Check sheet for the drawn part. Datum: minimum x, y, z corner. Units: mm. A direction names the side the tool comes from. Coordinates: 2 decimals unless noted, no trailing zeros. Write each loop counter-clockwise with the first axis right and the second up, starting at its lowest first coordinate (ties: lowest second). Pieces come first, ordered by that corner, then holes. Notation, with made-up numbers: (89.5, 6) -> (129.5, 6) arc R29 cw to (129.5, 37) -> close; hole circle Ø6 at (40, 83.5). An arc over 180 degrees is marked (long way). Answer in a Markdown table with one row per item. Add a question column.
Q1. Section check B-B, the plane y = 7. Record the boundary of the cut face in (x, z), and give its area (3 significant figures).
Q2. Gauge pin test, flat ends, axial feed: P1, Ø1, axis at y = 3, z = 22, coming from the +X side; P2, Ø3, axis at x = 6, z = 21.5, coming from the +Y side; P3, Ø0.8, axis at y = 7, z = 25.5, coming from the +X side; P4, Ø6, axis at x = 13.5, y = 10.5, coming from the +Z side. Record the tip position at first contact, or that the pin passes through.
Q3. Section check C-C, the plane x = 13. Record the boundary of the cut face in (y, z).
Q4. Section check D-D, the plane y = 9. Record the boundary of the cut face in (x, z), and give its area (3 significant figures).
Q5. Tool access check on the marked faces 1, 2 and 3. Record the directions out of +Z, -Z, +X, -X, +Y, -Y that give a thin tool (end or side, any length) a straight path to the whole face; none if there is none.
Q6. Thickness scan on line 1 (Y direction, x = 22.5, z = 14.25); line 2 (X direction, y = 5.75, z = 16.5); line 3 (Z direction, x = 16.25, y = 5). Record the ranges inside material, lowest first.
Q7. Section check A-A, the plane z = 25.75. Record the boundary of the cut face in (x, y), and give its area (3 significant figures).
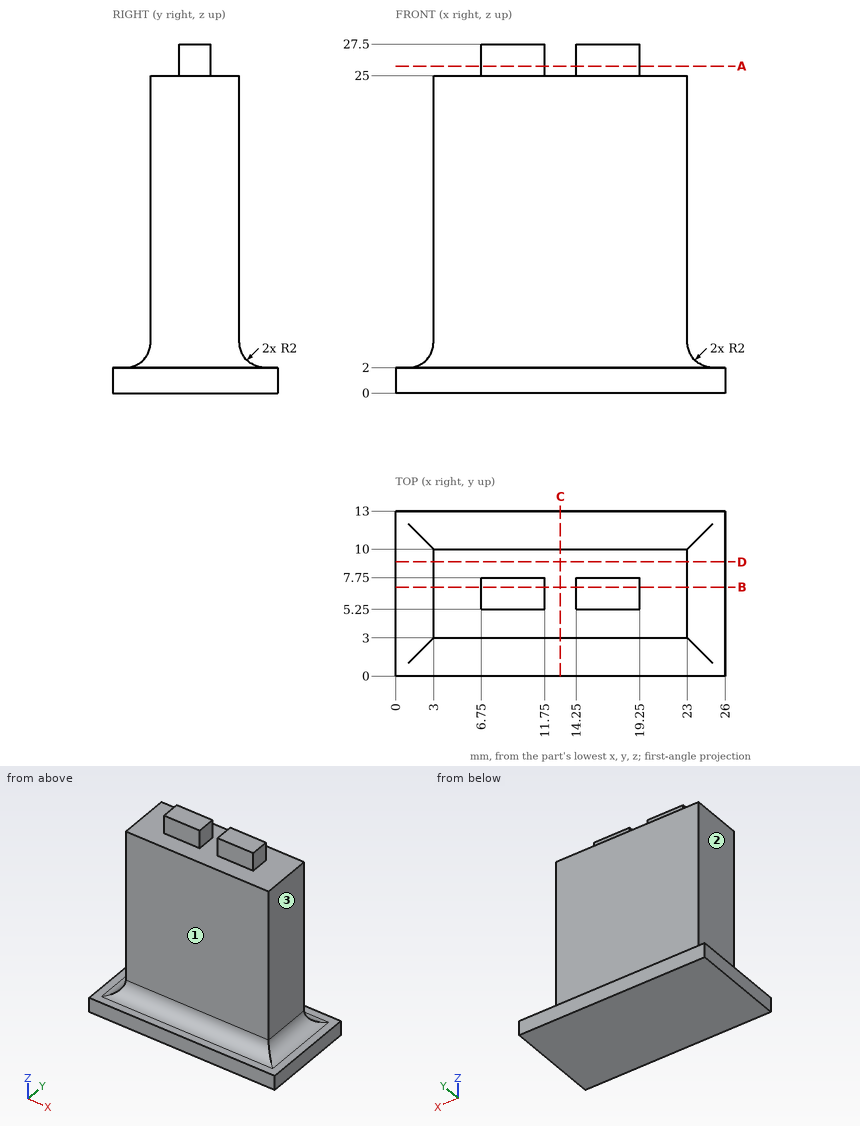
Calculated:
| question | item | result |
|---|---|---|
| 1 | outline | (0, 0) -> (26, 0) -> (26, 2) -> (25, 2) arc R2 cw to (23, 4) -> (23, 25) -> (19.25, 25) -> (19.25, 27.5) -> (14.25, 27.5) -> (14.25, 25) -> (11.75, 25) -> (11.75, 27.5) -> (6.75, 27.5) -> (6.75, 25) -> (3, 25) -> (3, 4) arc R2 cw to (1, 2) -> (0, 2) -> close |
| 1 | area | 539 mm² |
| 2 | P1 | stops at x = 23 |
| 2 | P2 | stops at y = 10 |
| 2 | P3 | stops at x = 19.25 |
| 2 | P4 | stops at z = 27.5 |
| 3 | outline | (0, 0) -> (13, 0) -> (13, 2) -> (12, 2) arc R2 cw to (10, 4) -> (10, 25) -> (3, 25) -> (3, 4) arc R2 cw to (1, 2) -> (0, 2) -> close |
| 4 | outline | (0, 0) -> (26, 0) -> (26, 2) -> (25, 2) arc R2 cw to (23, 4) -> (23, 25) -> (3, 25) -> (3, 4) arc R2 cw to (1, 2) -> (0, 2) -> close |
| 4 | area | 514 mm² |
| 5 | face 1 | +Z, +X, -X, -Y |
| 5 | face 2 | +Z, -X, +Y, -Y |
| 5 | face 3 | +Z, +X, +Y, -Y |
| 6 | line 1 | y = 3 to 10 |
| 6 | line 2 | x = 3 to 23 |
| 6 | line 3 | z = 0 to 25 |
| 7 | outline | (6.75, 5.25) -> (11.75, 5.25) -> (11.75, 7.75) -> (6.75, 7.75) -> close; (14.25, 5.25) -> (19.25, 5.25) -> (19.25, 7.75) -> (14.25, 7.75) -> close |
| 7 | area | 25.0 mm² |
